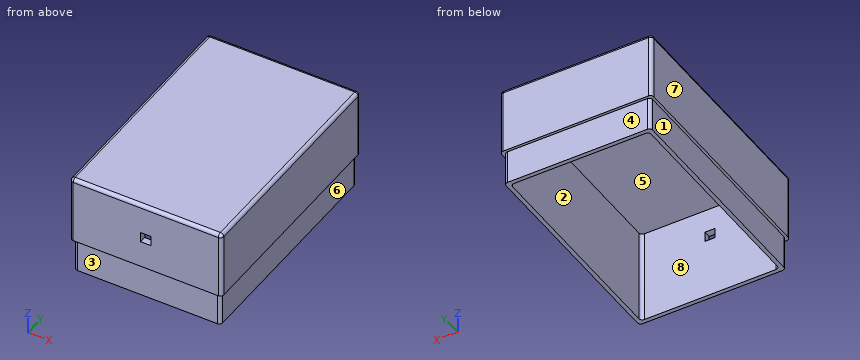
```python
from build123d import *

# Parameters (mm, degrees)
SKETCH011_W     = 45
SKETCH011_H     = 68
PAD007_DEPTH    = 2
SKETCH012_W     = 45
SKETCH012_H     = 68
SKETCH012_W_2   = 41
SKETCH012_H_2   = 64
PAD008_DEPTH    = 18
SKETCH013_W     = 43.4
SKETCH013_H     = 66.4
SKETCH013_W_2   = 41
SKETCH013_H_2   = 64
PAD009_DEPTH    = 10
SKETCH014_W     = 3
SKETCH014_H     = 3
POCKET004_DEPTH = 5
FILLET_R        = 1
FILLET002_R     = 1


with BuildPart() as part:
    # Sketch011 → Pad007 (new body)
    with BuildSketch(Plane.XY):
        Rectangle(SKETCH011_W, SKETCH011_H)
    extrude(amount=-PAD007_DEPTH)

    # Sketch012 (on Face6 of Pad007) → Pad008 (join)
    with BuildSketch(Plane(origin=(0, 0, -2), x_dir=(1, 0, 0), z_dir=(0, 0, -1))):
        Rectangle(SKETCH012_W, SKETCH012_H)
        Rectangle(SKETCH012_W_2, SKETCH012_H_2, mode=Mode.SUBTRACT)
    extrude(amount=PAD008_DEPTH)

    # Sketch013 (on Face9 of Pad008) → Pad009 (join)
    with BuildSketch(Plane(origin=(0, 0, -20), x_dir=(1, 0, 0), z_dir=(0, 0, -1))):
        Rectangle(SKETCH013_W, SKETCH013_H)
        Rectangle(SKETCH013_W_2, SKETCH013_H_2, mode=Mode.SUBTRACT)
    extrude(amount=PAD009_DEPTH)

    # Sketch014 (on Face10 of Pad009) → Pocket004 (cut)
    with BuildSketch(Plane.XZ.offset(34)):
        with Locations((0, -10.5)):
            Rectangle(SKETCH014_W, SKETCH014_H)
    extrude(amount=-POCKET004_DEPTH, mode=Mode.SUBTRACT)

    # Fillet
    fillet_edges = [part.edges().sort_by_distance(p)[0] for p in [
        (-22.5, 0, 0),
        (0, 34, 0),
        (22.5, 0, 0),
        (0, -34, 0),
        (-22.5, -34, -11),
        (-22.5, 34, -11),
        (22.5, -34, -11),
        (22.5, 34, -11),
    ]]
    fillet(fillet_edges, radius=FILLET_R)

    # Fillet002
    fillet002_edges = [part.edges().sort_by_distance(p)[0] for p in [
        (-20.5, -32, -25),
        (-21.7, -33.2, -25),
        (21.7, -33.2, -25),
        (20.5, -32, -25),
        (21.7, 33.2, -25),
        (20.5, 32, -25),
        (-21.7, 33.2, -25),
        (-20.5, 32, -25),
    ]]
    fillet(fillet002_edges, radius=FILLET002_R)


with BuildPart() as part_1:
    # Body002 placement: moved
    add(part.part.moved(Location((0, 0, 21))))


solid = part_1.part
```
The model under review builds one solid part; all positions refer to its coordinate system, in mm. Face numbers are marked on the shaded views. A direction names the side the tool comes from. Round coordinates to 2 decimals unless told otherwise and drop trailing zeros. Loops run counter-clockwise (first coordinate to the right, second up) from the corner with the lowest first, then second, coordinate; pieces in that order, holes last. Notation, with made-up numbers: (18, -26) -> (34, -26) arc R17 cw to (34, -7) -> close; hole circle Ø5 at (21.25, 25.5). An arc over 180 degrees is marked (long way). Answer as a JSON object with one key per item and string values. Group by question number.
1) We need section C-C on x = 6. Write out the cut boundary in (y, z), then the cut area to 3 significant figures.
2) For pin 1 Ø0.6 at (y, z) = (-33.5, 11) entering from -X; pin 2 Ø5 at (x, z) = (3.5, -4.5) entering from -Y; pin 3 Ø5 at (y, z) = (4.5, -2) entering from -X, all flat-tipped, find the tip position at first contact; note any pin that passes through.
3) Mouldability with a two-part tool opening along X and no side actions: class the marked faces 5, 6, 7 and 8 as released by +X, released by -X, zero draft, split by the parting line, or undercut.
4) For the marked faces 1, 2, 3 and 4, list the 3-axis set-ups (+Z, -Z, +X, -X, +Y, -Y) from which the entire face can be reached by the end or side of a thin tool; tool diameter is ignored.
5) For line 1 (Y direction, x = 16.5, z = 2.25); line 2 (X direction, y = -10, z = 3); line 3 (X direction, y = 18, z = -4.5), list the stretches that pass through material, from the lowest coordinate up. Write a range as [from, to].
6) We need section B-B on y = 23. Write out the cut boundary in (x, z).
7) We need section A-A on z = 8.25. Write out the cut boundary in (x, y).
Result set:
{
 "1": {"outline": "(-34, 1) -> (-33.2, 1) -> (-33.2, -9) -> (-32, -9) -> (-32, 19) -> (32, 19) -> (32, -9) -> (33.2, -9) -> (33.2, 1) -> (34, 1) -> (34, 20) arc R1 ccw to (33, 21) -> (-33, 21) arc R1 ccw to (-34, 20) -> close", "area": "232 mm²"},
 "2": {"pin 1": "x = -22.48", "pin 2": "y = -33.2", "pin 3": "x = -21.7"},
 "3": {"face 5": "undercut", "face 6": "released by +X", "face 7": "released by -X", "face 8": "undercut"},
 "4": {"face 1": "-Z, -X, +Y, -Y", "face 2": "-Z", "face 3": "-Z, +X, -X, -Y", "face 4": "-Z, +X, -X, +Y"},
 "5": {"line 1": "[-34, -32], [32, 34]", "line 2": "[-22.5, -20.5], [20.5, 22.5]", "line 3": "[-21.7, -20.5], [20.5, 21.7]"},
 "6": {"outline": "(-22.5, 1) -> (-21.7, 1) -> (-21.7, -9) -> (-20.5, -9) -> (-20.5, 19) -> (20.5, 19) -> (20.5, -9) -> (21.7, -9) -> (21.7, 1) -> (22.5, 1) -> (22.5, 20) arc R1 ccw to (21.5, 21) -> (-21.5, 21) arc R1 ccw to (-22.5, 20) -> close"},
 "7": {"outline": "(-22.5, -33) arc R1 ccw to (-21.5, -34) -> (21.5, -34) arc R1 ccw to (22.5, -33) -> (22.5, 33) arc R1 ccw to (21.5, 34) -> (-21.5, 34) arc R1 ccw to (-22.5, 33) -> close; hole (-20.5, -31) arc R1 ccw to (-19.5, -32) -> (19.5, -32) arc R1 ccw to (20.5, -31) -> (20.5, 31) arc R1 ccw to (19.5, 32) -> (-19.5, 32) arc R1 ccw to (-20.5, 31) -> close"}
}
